The listing builds one solid part. Answer for the finished solid, in the listing's coordinates (mm). A direction names the side the tool comes from. Give positions to 0.01 mm unless a question says otherwise; leave off trailing zeros. Loops run counter-clockwise (first coordinate to the right, second up) from the corner with the lowest first, then second, coordinate; pieces in that order, holes last. Notation, with made-up numbers: M 81.5,29 L 125.5,29 A24 cw 125.5,64 Z; hole C 35.5,68 d2. An arc over 180 degrees is marked long. Use one line per item in the form item = value. Start each with the question number.
1. The part is cut by section B-B (x = 2). Write down the section's boundary in (y, z).
2. For faces 4 (the face through (2.6, 9, 3)), 5 (the face through (-2, 1, 6.25)), 6 (the face through (-3, -1.8, 2)), 7 (the face through (3.43, 0.91, 3.08)), 8 (the face through (0, 7.35, 6)), determine the directions among +Z, -Z, +X, -X, +Y, -Y from which every point of the face is accessible in a straight line to the end or side of a thin tool.
3. The part is cut by section D-D (z = 1.75). Write down the section's boundary in (x, y), and give its area (3 significant figures).
4. The part is cut by section C-C (y = 5.75). Write down the section's boundary in (x, z), and give its area (3 significant figures).
5. Straight lines are drawn through the part: line 1 (Y direction, x = -1.5, z = 6.75); line 2 (X direction, y = 2, z = 1.75); line 3 (Y direction, x = -1.5, z = 6). For each, find the intervals that lie inside material, in ascending order. Write a range as from..to.
6. Each of these flat-tipped pins is pushed along its axis until it touches: pin 1 Ø1.1 at (x, y) = (2.5, 1) entering from +Z; pin 2 Ø2 at (y, z) = (8.5, 2) entering from +X; pin 3 Ø1.8 at (y, z) = (13, 6.5) entering from -X. Where does it stop, or does it pass through?
7. The mould has two halves that part along Y. Classify faces 1 (the face through (2, -3.2, 2)), 2 (the face through (-2, -2, 5)), 3 (the face through (-1, 10.65, 6)): released by +Y, released by -Y, zero draft, split by the parting line, or undercut.
8. The part is cut by section A-A (z = 6). Write down the section's boundary in (x, y).
from build123d import *

# Parameters (mm, degrees)
PAD017_DEPTH           = 5
PAD020_DEPTH           = 6.25
SKETCH055_W            = 5.2
SKETCH055_H            = 1.65
PAD025_DEPTH           = 7.5
SKETCH052_W            = 5.2
SKETCH052_H            = 1.65
PAD026_DEPTH           = 4.6
SKETCH053_W            = 2.1
SKETCH053_H            = 1.65
PAD027_DEPTH           = 7.5
SKETCH054_W            = 5.2
SKETCH054_H            = 1.65
PAD028_DEPTH           = 7.5
LINEARPATTERN011_COUNT = 2
LINEARPATTERN011_PITCH = 3.3
CHAMFER001_SIZE        = 1


with BuildPart() as obj1:
    # Sketch034 → Pad017 (new body)
    with BuildSketch(Plane.XY):
        with BuildLine():
            Line((-1.35, -1.8), (-1.35, 6))
            ThreePointArc((0, 7.35), (-0.954594, 6.954594), (-1.35, 6))
            Line((0, 9), (0, 7.35))
            Line((-2.6, 9), (0, 9))
            Line((-2.6, -1.8), (-2.6, 9))
            Line((-3.85, -1.8), (-2.6, -1.8))
            ThreePointArc((-3.85, -1.8), (-3.439949, -2.789949), (-2.45, -3.2))
            Line((-1.35, -3.2), (-2.45, -3.2))
            Line((-1.35, -1.8), (-1.35, -3.2))
        make_face()
    extrude(amount=PAD017_DEPTH)

    # Sketch037 → Pad020 (join)
    with BuildSketch(Plane.XY):
        Polygon((-1.35, 0.2), (-1.35, 1.6), (-2.6, 1.6), (-3.85, 1.6), (-3, 0.2), (-2.6, 0.2), align=None)
    extrude(amount=PAD020_DEPTH)


with BuildPart() as obj2:
    # Mirror001: instance of _obj1
    add(obj1.part.mirror(Plane(origin=(0, 0, 0), x_dir=(0, 1, 0), z_dir=(-1, 0, 0))))


with BuildPart() as body018:
    # Fusion001 base: copy of _obj1
    add(obj1.part)

    # Fusion001: union _obj2)
    add(obj2.part)

    # Sketch055 → Pad025 (new body)
    with BuildSketch(Plane.XY):
        with Locations((0, 8.175)):
            Rectangle(SKETCH055_W, SKETCH055_H)
    extrude(amount=PAD025_DEPTH)

    # Sketch052 → Pad026 (join)
    with BuildSketch(Plane.XY):
        with Locations((0, 9.825)):
            Rectangle(SKETCH052_W, SKETCH052_H)
    pad026 = extrude(amount=PAD026_DEPTH)

    # Sketch053 → Pad027 (join)
    with BuildSketch(Plane.XY):
        with Locations((1.55, 9.825)):
            Rectangle(SKETCH053_W, SKETCH053_H)
    pad027 = extrude(amount=PAD027_DEPTH)

    # Sketch054 → Pad028 (join)
    with BuildSketch(Plane.XY):
        with Locations((0, 11.475)):
            Rectangle(SKETCH054_W, SKETCH054_H)
    pad028 = extrude(amount=PAD028_DEPTH)

    # LinearPattern011: Pad026, Pad027, Pad028 ×2
    with Locations(*[(0, i * LINEARPATTERN011_PITCH, 0) for i in range(1, LINEARPATTERN011_COUNT)]):
        add(pad026)
        add(pad027)
        add(pad028)

    # Chamfer001
    chamfer001_edges = [body018.edges().sort_by_distance(p)[0] for p in [
        (-2.6, 14.775, 7.5),
        (-2.6, 11.475, 7.5),
        (-2.6, 8.175, 7.5),
    ]]
    chamfer(chamfer001_edges, length=CHAMFER001_SIZE)


solid = body018.part
Derived:
q1.outline = M -3.2,0 L 15.6,0 L 15.6,7.5 L 7.35,7.5 L 7.35,5 L 1.6,5 L 1.6,6.25 L 0.2,6.25 L 0.2,5 L -3.2,5 Z
q2.face_4 = +Z, -Z, +X, +Y
q2.face_5 = +Z, +X, -X, -Y
q2.face_6 = +Z, -Z, -X
q2.face_7 = +Z, -Z, +X
q2.face_8 = +Z, +X, -X
q3.outline = M -3.85,-1.8 A1.4 ccw -2.45,-3.2 L -1.35,-3.2 L -1.35,6 A1.35 cw 0,7.35 A1.35 cw 1.35,6 L 1.35,-3.2 L 2.45,-3.2 A1.4 ccw 3.85,-1.8 L 2.6,-1.8 L 2.6,0.2 L 3,0.2 L 3.85,1.6 L 2.6,1.6 L 2.6,15.6 L -2.6,15.6 L -2.6,1.6 L -3.85,1.6 L -3,0.2 L -2.6,0.2 L -2.6,-1.8 Z
q3.area = 75.0 mm2
q4.outline = M -2.6,0 L -1.35,0 L -1.35,5 L -2.6,5 Z; M 1.35,0 L 2.6,0 L 2.6,5 L 1.35,5 Z
q4.area = 12.5 mm2
q5.line_1 = 7.35..9, 10.65..12.3, 13.95..15.6
q5.line_2 = -2.6..-1.35, 1.35..2.6
q5.line_3 = 0.2..1.6, 7.35..9, 10.65..12.3, 13.95..15.6
q6.pin_1 = 6.25
q6.pin_2 = 2.6
q6.pin_3 = -2.6
q7.face_1 = released by -Y
q7.face_2 = zero draft
q7.face_3 = undercut
q8.outline = M -3.85,1.6 L -3,0.2 L -1.35,0.2 L -1.35,1.6 Z; M -2.6,7.35 L 2.6,7.35 L 2.6,15.6 L -2.6,15.6 L -2.6,13.95 L 0.5,13.95 L 0.5,12.3 L -2.6,12.3 L -2.6,10.65 L 0.5,10.65 L 0.5,9 L -2.6,9 Z; M 1.35,0.2 L 3,0.2 L 3.85,1.6 L 1.35,1.6 Z
